Design review of the part shown in the three views and the two pictorial views. Dimensions are in mm from the part's minimum x, y and z. A direction names the side the tool comes from. Give positions to 0.01 mm unless a question says otherwise; leave off trailing zeros. Loops run counter-clockwise (first coordinate to the right, second up) from the corner with the lowest first, then second, coordinate; pieces in that order, holes last. Notation, with made-up numbers: (22, 34.25) - (66, 34.25) arc R23 ccw to (66, 55.25) - close; hole circle Ø11 at (-23, -20). An arc over 180 degrees is marked (long way). Return JSON: item names as keys, results as strings. Group by question number.
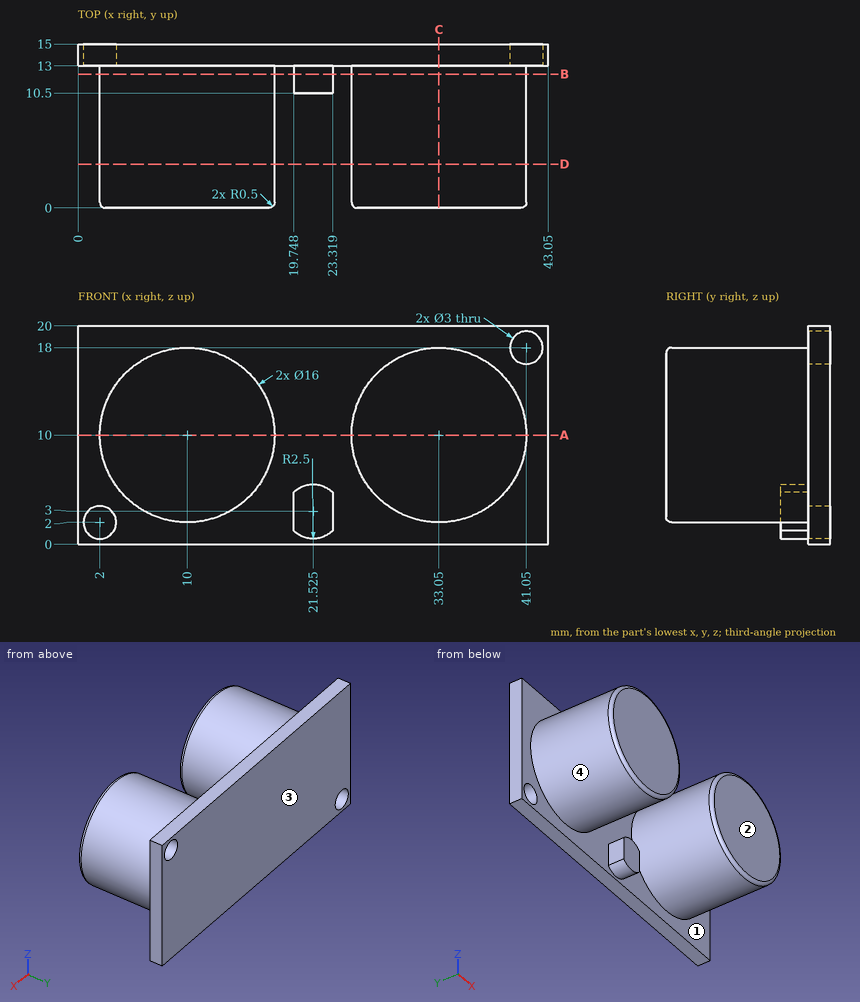
Item 1: For L1, parallel to X at y = 14.5, z = 2; L2, parallel to X at y = 14.6, z = 18; L3, parallel to Z at x = 41.05, y = 13.8, list the stretches that pass through material, from the lowest coordinate up. Write a range as from..to.
Item 2: Mouldability with a two-part tool opening along X and no side actions: class the marked faces 1 and 2 as +X half, -X half, draft (parallel to the pull), parting line (faces both ways), or undercut.
Item 3: Tool access review of the marked faces 3 and 4: name each direction out of +Z, -Z, +X, -X, +Y, -Y from which nothing blocks a thin tool from reaching the whole face with its end or side.
Item 4: Take a section at D-D (y = 4). State the section outline as (x, z) points, then the cut area to 3 significant figures.
Item 5: For P1, Ø6, axis at y = 2, z = 5.5, coming from the -X side; P2, Ø2, axis at y = 11.5, z = 7, coming from the +X side; P3, Ø2, axis at y = 11.5, z = 3.5, coming from the +X side, all flat-tipped, find the tip position at first contact; note any pin that passes through.
Item 6: Take a section at B-B (y = 12.25). State how many separate pieces and enclosed holes the cut face has, then the cut area to 3 significant figures.
Item 7: Take a section at A-A (z = 10). State the section outline as (x, y) points.
Item 8: Take a section at C-C (x = 33.05). State the section outline as (y, z) points, then the cut area to 3 significant figures.
Check sheet entries:
{
 "1": {"L1": "x = 0..0.5, 3.5..43.05", "L2": "x = 0..39.55, 42.55..43.05", "L3": "z = 0..16.5, 19.5..20"},
 "2": {"face 1": "undercut", "face 2": "draft"},
 "3": {"face 3": "+Z, -Z, +X, -X, +Y", "face 4": "-Y"},
 "4": {"outline": "circle Ø16 at (10, 10); circle Ø16 at (33.05, 10)", "area": "402 mm^2"},
 "5": {"P1": "stops at x = 2.14", "P2": "stops at x = 40.8", "P3": "stops at x = 38.86"},
 "6": {"separate pieces": "3", "enclosed holes": "0", "area": "418 mm^2"},
 "7": {"outline": "(0, 13) - (2, 13) - (2, 0.5) arc R0.5 ccw to (2.5, 0) - (17.5, 0) arc R0.5 ccw to (18, 0.5) - (18, 13) - (25.05, 13) - (25.05, 0.5) arc R0.5 ccw to (25.55, 0) - (40.55, 0) arc R0.5 ccw to (41.05, 0.5) - (41.05, 13) - (43.05, 13) - (43.05, 15) - (0, 15) - close"},
 "8": {"outline": "(0, 2.5) arc R0.5 ccw to (0.5, 2) - (13, 2) - (13, 0) - (15, 0) - (15, 20) - (13, 20) - (13, 18) - (0.5, 18) arc R0.5 ccw to (0, 17.5) - close", "area": "248 mm^2"}
}
